Autodesk Inventor part; units mm, degrees
ref_plane "YZ Plane" through (0, 0, 0) normal (1, 0, 0) x (0, 1, 0)
ref_plane "XZ Plane" through (0, 0, 0) normal (0, 1, 0) x (-1, 0, 0)
ref_plane "XY Plane" through (0, 0, 0) normal (0, 0, 1) x (1, 0, 0)
sketch "Sketch1" plane through (0, 0, 0) normal (0, 0, 1) x (1, 0, 0)
  circle A0 centre (0, 0) radius 14.2875
  circle A1 centre (0, 0) radius 20.6375
  line L0 (20.6375, -241.3) -> (-20.6375, -241.3)
  line L1 (-20.6375, 0) -> (-20.6375, -241.3)
  line L2 (20.6375, -241.3) -> (20.6375, 0)
  dimension "d0" = 28.575
  dimension "d1" = 6.35
  dimension "d2" = 241.3
extrude "Extrusion1" add sketch "Sketch1" along normal mid plane 6.35
properties part number "CL2-001" material "Aluminum 6061"
Geometry: final body of the model. Coordinates: model frame, mm. Round coordinates to 2 decimals unless told otherwise and drop trailing zeros. Loops run counter-clockwise (first coordinate to the right, second up) from the corner with the lowest first, then second, coordinate; pieces in that order, holes last.
Q1. Section A-A on x = 0. Return loops of the section in (y, z) (1 decimal).
Q2. Section C-C on x = -16.5. Return loops of the section in (y, z) (3 decimals), plus the area to 3 significant figures.
Q3. Section B-B on z = 1.25. Return loops of the section in (x, y) (1 decimal).
Q4. Material intervals for L1, parallel to Y at x = 0, z = -1; L2, parallel to Y at x = -9, z = 0.75, sorted ascending.
Q5. Pin query (flat end, axial travel): P1, Ø3, axis at x = 14, z = 1, coming from the +Y side. Return the tip coordinate at first contact, or that it passes through.
Q6. Pull-direction query (X, two-part tool) for faces 1 (the flat face through (20.638, -122, 0)), 2 (the flat face through (0, -108, -3.175)), 3 (the cylindrical face through (-14.274, -0.628, -0.044)), 4 (the flat face through (-20.638, -119, 0)); classes: released by +X, released by -X, zero draft, split by the parting line, or undercut.
Evaluation:
1. outline: (-241.3, -3.2) - (-14.3, -3.2) - (-14.3, 3.2) - (-241.3, 3.2) - close; (14.3, -3.2) - (20.6, -3.2) - (20.6, 3.2) - (14.3, 3.2) - close
2. outline: (-241.3, -3.175) - (12.396, -3.175) - (12.396, 3.175) - (-241.3, 3.175) - close
2. area: 1,610 mm2
3. outline: (-20.6, -241.3) - (20.6, -241.3) - (20.6, 0) arc R20.6 ccw to (-20.6, 0) - close; hole circle Ø28.6 at (0, 0)
4. L1: y = -241.3 to -14.29, 14.29 to 20.64
4. L2: y = -241.3 to -11.1, 11.1 to 18.57
5. P1: stops at y = 16.42
6. face 1: released by +X
6. face 2: zero draft
6. face 3: undercut
6. face 4: released by -X
